from build123d import *
from build123d.topology import SkipClean

# Parameters (mm, degrees)
SKETCH1_R           = 50.8
BOSS_EXTRUDE1_DEPTH = 50.8
SKETCH2_R           = 44.45
CUT_EXTRUDE1_DEPTH  = 44.45
BOSS_EXTRUDE2_START = 76.2
BOSS_EXTRUDE2_DEPTH = 76.2
BOSS_EXTRUDE3_START = 1.905
BOSS_EXTRUDE3_DEPTH = 1.905


with BuildPart() as part:
    # Sketch1 → Boss-Extrude1 (new body)
    with BuildSketch(Plane.XY):
        Circle(SKETCH1_R)
    extrude(amount=BOSS_EXTRUDE1_DEPTH)

    # Sketch2 → Cut-Extrude1 (cut)
    with BuildSketch(Plane(origin=(0, 0, 0), x_dir=(-1, 0, 0), z_dir=(0, 0, -1))):
        Circle(SKETCH2_R)
    extrude(amount=-CUT_EXTRUDE1_DEPTH, mode=Mode.SUBTRACT)

    # Sketch3 → Boss-Extrude2 (add)
    with BuildSketch(Plane(origin=(0, 0, 0), x_dir=(-1, 0, 0), z_dir=(0, 0, -1)).offset(BOSS_EXTRUDE2_START)):
        with BuildLine():
            Line((-36.278456417, -35.56), (-26.67, -35.56))
            ThreePointArc((-26.67, -35.56), (31.430896424, -31.430896424), (35.56, 26.67))
            Line((35.56, 26.67), (35.56, 36.278456417))
            ThreePointArc((35.56, 36.278456417), (35.921024484, -35.921024484), (-36.278456417, -35.56))
        make_face()
    extrude(amount=-BOSS_EXTRUDE2_DEPTH)

    # Sketch4 → Boss-Extrude3 (add)
    with SkipClean():  # the faces are left unmerged after this step: merging them gives an invalid solid
        with BuildSketch(Plane(origin=(0, 0, 0), x_dir=(-1, 0, 0), z_dir=(0, 0, -1)).offset(BOSS_EXTRUDE3_START)):
            with BuildLine():
                Line((-46.558969061, -20.32), (-39.533531337, -20.32))
                ThreePointArc((-39.533531337, -20.32), (-31.430896424, 31.430896424), (20.32, 39.533531337))
                Line((20.32, 39.533531337), (20.32, 46.558969061))
                ThreePointArc((20.32, 46.558969061), (-35.921024484, 35.921024484), (-46.558969061, -20.32))
            make_face()
        extrude(amount=-BOSS_EXTRUDE3_DEPTH)


solid = part.part
Geometry check sheet. Reference: the model listing, model coordinates, mm. A direction names the side the tool comes from. Give positions to 0.01 mm unless a question says otherwise; leave off trailing zeros. Write each loop counter-clockwise with the first axis right and the second up, starting at its lowest first coordinate (ties: lowest second). Pieces come first, ordered by that corner, then holes. Notation, with made-up numbers: (-1.5, 17.25) - (7.5, 17.25) arc R25 cw to (7.5, 52.25) - close; hole circle Ø8 at (75.25, -31). An arc over 180 degrees is marked (long way). Put each result on its own line as item: value.
1. Set-up check for faces 1 (the flat face through (34, 31, -1.905)), 2 (the flat face through (-1, 1, 50.8)): record each of +Z, -Z, +X, -X, +Y, -Y from which the full face is reachable in a straight line by a thin tool's end or side.
Ans:
face 1: -Z, +X, +Y
face 2: +Z, +X, -X, +Y, -Y
2. Draft check along Y on faces 3 (the flat face through (-28, 37, 0)), 4 (the flat face through (1, 1, 44.45)), 5 (the flat face through (39, -28, 0)). Enter one of: +Y half, -Y half, draft (parallel to the pull), parting line (faces both ways), or undercut.
Ans:
face 3: draft
face 4: undercut
face 5: undercut
3. Thickness scan on line 1 (Y direction, x = 0, z = 11.5); line 2 (Z direction, x = -28.5, y = 17.5). Record the ranges inside material, lowest first.
Ans:
line 1: y = -50.8 to -44.45, 44.45 to 50.8
line 2: z = 44.45 to 50.8
4. Sectioned sample at A-A, the plane y = 0. Enter the section's corners in (x, z) (3 decimals), plus the area to 3 significant figures.
Ans:
outline: (-50.8, -76.2) - (-44.45, -76.2) - (-44.45, 44.45) - (44.45, 44.45) - (44.45, -1.905) - (50.8, -1.905) - (50.8, 50.8) - (-50.8, 50.8) - close
area: 1,710 mm²
5. Sectioned sample at C-C, the plane z = 31.5. Enter the section's corners in (x, y).
Ans:
outline: circle Ø101.6 at (0, 0); hole circle Ø88.9 at (0, 0)
6. Go/stop test with flat-tipped pins: pin 1 (12 mm diameter, centred on x = -28.5, y = 41, fed in from -Z); pin 2 (2 mm diameter, centred on x = -33.5, z = 6, fed in from -Y); pin 3 (2 mm diameter, centred on x = -8.5, z = -62.5, fed in from -Y). Record where each tip stops, or that it passes through.
Ans:
pin 1: stops at z = 0
pin 2: stops at y = -39.04
pin 3: stops at y = -50.24
